from build123d import *

# Parameters (mm, degrees)
F0_R     = 3.59
F1_DEPTH = 3.67
F3_DEPTH = 3.671
F4_W     = 6.9088
F4_H     = 18.185156
F4_W_2   = 6.909577
F5_DEPTH = 3.671


with BuildPart() as f1:
    # F0 (on Front) → F1 (new body)
    with BuildSketch(Plane.XZ):
        with BuildLine():
            Line((-46.744851, 19.260988), (-46.744851, 10.16))
            Line((-46.744851, 10.16), (-46.744851, 0))
            Line((-46.744851, 0), (-38.524851, 0))
            Line((-38.524851, 0), (-38.524851, 10.16))
            Line((-38.524851, 10.16), (-28.284851, 10.16))
            Line((-28.284851, 10.16), (-28.284851, 0))
            Line((-28.284851, 0), (-20.064851, 0))
            Line((-20.064851, 0), (-20.064851, 10.16))
            Line((-20.064851, 10.16), (-20.064851, 19.260988))
            ThreePointArc((-20.064851, 19.260988), (-21.924723, 23.751116), (-26.414851, 25.610988))
            Line((-26.414851, 25.610988), (-40.394851, 25.610988))
            ThreePointArc((-40.394851, 25.610988), (-44.884979, 23.751116), (-46.744851, 19.260988))
        make_face()
        with Locations((-33.377483, 16.686028)):
            Circle(F0_R, mode=Mode.SUBTRACT)
    extrude(amount=F1_DEPTH)

    # F2 (on face) → F3 (cut, through all)
    with BuildSketch(Plane.XZ.offset(3.67)):
        with BuildLine():
            ThreePointArc((-53.653651, 34.695156), (-51.793779, 30.205028), (-47.303651, 28.345156))
            Line((-47.303651, 28.345156), (-4.503874, 28.345156))
            Line((-4.503874, 28.345156), (-4.503874, 41.061975))
            Line((-4.503874, 41.061975), (-53.653651, 41.061975))
            Line((-53.653651, 41.061975), (-53.653651, 34.695156))
        make_face()
    extrude(amount=-F3_DEPTH, mode=Mode.SUBTRACT)

    # F4 (on face) → F5 (cut, through all)
    with BuildSketch(Plane.XZ.offset(3.67)):
        with Locations((-50.199251, 9.092578)):
            Rectangle(F4_W, F4_H)
        with Locations((-16.610062, 9.092578)):
            Rectangle(F4_W_2, F4_H)
    extrude(amount=-F5_DEPTH, mode=Mode.SUBTRACT)


solid = f1.part
Input: part model. Units: mm. Frame: model coordinates. A direction names the side the tool comes from. Coordinates: 2 decimals unless noted, no trailing zeros. Loops run counter-clockwise (first coordinate to the right, second up) from the corner with the lowest first, then second, coordinate; pieces in that order, holes last.
(1) Section A-A on z = 8. Return the cut outline in (x, y).
(2) Pull-direction query (X, two-part tool) for faces 3 (the face through (-46.745, -2, 10)), 4 (the face through (-29.95, -1.81, 17.76)), 5 (the face through (-33, -2, 10.16)), 6 (the face through (-24, -2, 0)); classes: released by +X, released by -X, zero draft, split by the parting line, or undercut.
(3) Material intervals for probe 1 along X at (y, z) = (-1.2, 1.5); probe 2 along Z at (x, y) = (-33.25, -0.75); probe 3 along Z at (x, y) = (-32, -1), sorted ascending.
(4) Section C-C on y = -1.15. Return the cut outline in (x, z), then the cut area to 3 significant figures.
(5) Set-up query: faces 1 (the face through (-44.835, -1.809, 23.8)), 2 (the face through (-38.525, -2, 5)). Return all of +Z, -Z, +X, -X, +Y, -Y with unobstructed straight access to the full face (end or side cutting, diameter ignored); none if empty.
(6) Section B-B on x = -34.5. Return the cut outline in (y, z).
(7) Section D-D on x = -42.75. Return the cut outline in (y, z), then the cut area to 3 significant figures.
(8) First-contact query: pin 1 Ø11.5 at (x, z) = (-33.38, 16.69) entering from +Y. Flat tip, straight axial feed; report the tip coordinate or a pass-through.
Data:
1. outline: (-46.74, -3.67) - (-38.52, -3.67) - (-38.52, 0) - (-46.74, 0) - close; (-28.28, -3.67) - (-20.06, -3.67) - (-20.06, 0) - (-28.28, 0) - close
2. face 3: released by -X
2. face 4: undercut
2. face 5: undercut
2. face 6: zero draft
3. probe 1: x = -46.74 to -38.52, -28.28 to -20.06
3. probe 2: z = 10.16 to 13.1, 20.27 to 25.61
3. probe 3: z = 10.16 to 13.37, 20 to 25.61
4. outline: (-46.74, 0) - (-38.52, 0) - (-38.52, 10.16) - (-28.28, 10.16) - (-28.28, 0) - (-20.06, 0) - (-20.06, 19.26) arc R6.35 ccw to (-26.41, 25.61) - (-40.39, 25.61) arc R6.35 ccw to (-46.74, 19.26) - close; hole circle Ø7.18 at (-33.38, 16.69)
4. area: 521 mm2
5. face 1: +Z, -X, +Y, -Y
5. face 2: -Z, +Y, -Y
6. outline: (-3.67, 10.16) - (0, 10.16) - (0, 13.28) - (-3.67, 13.28) - close; (-3.67, 20.1) - (0, 20.1) - (0, 25.61) - (-3.67, 25.61) - close
7. outline: (-3.67, 0) - (0, 0) - (0, 25.16) - (-3.67, 25.16) - close
7. area: 92.3 mm2
8. pin 1: stops at y = 0
